CAD build for the part. Positions are in the model's coordinates, mm. A direction names the side the tool comes from. Coordinates: 2 decimals unless noted, no trailing zeros. Loops run counter-clockwise (first coordinate to the right, second up) from the corner with the lowest first, then second, coordinate; pieces in that order, holes last.
1) Saw through at A-A, the plane y = 0. Write the cut outline in (x, z).
2) Which spindle directions (+Z, -Z, +X, -X, +Y, -Y) get a long thin tool onto all of the face, cutting with end or side? Do faces 1 (the cylindrical face through (46.99, -47.15, 50.56)), 2 (the flat face through (-47.465, 0.25, 21.554)). Say none if no direction does.
3) Saw through at B-B, the plane x = 0. Write the cut outline in (y, z).
4) Saw through at C-C, the plane z = 73.5. Write the cut outline in (x, y), and give its area (3 significant figures).
5) Two-plate mould, pull along Z, no slides. Class faces 3 (the flat face through (-38, 0, 24.019)), 4 (the cylindrical face through (-47.15, 0.56, 3.01)), 5 (the cylindrical face through (-46.99, 0.56, 97.15)): +Z half, -Z half, draft (parallel to the pull), parting line (faces both ways), or undercut.
6) Pin check, flat tips, straight feed: pin 1 Ø15.5 at (y, z) = (-3.5, 53) entering from -X; pin 2 Ø15 at (x, y) = (9, -2) entering from +Z. Stop position of each tip, or through.
7) Wall check: line 1 along Y through (x, z) = (0, 84.75); line 2 along Z through (x, y) = (-30, -40.5); line 3 along X through (y, z) = (-15.5, 92.5). Give the ranges that are in metal, low to high.
```python
from build123d import *

# Parameters (mm, degrees)
SKETCH1_W           = 100
SKETCH1_H           = 100
BOSS_EXTRUDE1_DEPTH = 100
SKETCH2_R           = 25
CUT_EXTRUDE1_DEPTH  = 20
CUT_EXTRUDE3_DEPTH  = 20
CHAMFER1_SIZE       = 5
FILLET1_R           = 10
FILLET2_R           = 10
FILLET3_R           = 10


with BuildPart() as part:
    # Sketch1 → Boss-Extrude1 (new body)
    with BuildSketch(Plane.XY):
        Rectangle(SKETCH1_W, SKETCH1_H)
    extrude(amount=BOSS_EXTRUDE1_DEPTH)

    # Sketch2 → Cut-Extrude1 (cut)
    with BuildSketch(Plane.XY.offset(100)):
        Circle(SKETCH2_R)
    extrude(amount=-CUT_EXTRUDE1_DEPTH, mode=Mode.SUBTRACT)

    # Sketch6 → Cut-Extrude3 (cut)
    with BuildSketch(Plane.ZY.offset(50)):
        Polygon((69.019237886, -19.019237886), (30.980762114, 19.019237886), (24.019237886, 15), (24.019237886, -15), (50, -30), align=None)
        Polygon((50, 30), (30.980762114, 19.019237886), (69.019237886, -19.019237886), (75.980762114, -15), (75.980762114, 15), align=None)
    extrude(amount=-CUT_EXTRUDE3_DEPTH, mode=Mode.SUBTRACT)

    # Chamfer1
    chamfer1_edges = [part.edges().sort_by_distance(p)[0] for p in [
        (-50, -22.5, 37.009618943),
        (-50, -22.5, 62.990381057),
        (-50, 0, 75.980762114),
        (-50, 22.5, 62.990381057),
        (-50, 22.5, 37.009618943),
        (-50, 0, 24.019237886),
    ]]
    chamfer(chamfer1_edges, length=CHAMFER1_SIZE)

    # Fillet1
    fillet1_edges = [part.edges().sort_by_distance(p)[0] for p in [
        (-25, 0, 100),
    ]]
    fillet(fillet1_edges, radius=FILLET1_R)

    # Fillet2
    fillet2_edges = [part.edges().sort_by_distance(p)[0] for p in [
        (-50, 0, 100),
        (0, -50, 100),
        (0, -50, 0),
        (50, -50, 50),
        (-50, -50, 50),
        (-50, 50, 50),
        (0, 50, 100),
    ]]
    fillet(fillet2_edges, radius=FILLET2_R)

    # Fillet3
    # the kernel refuses this fillet: 10 mm, written as the material it takes off along each edge
    with BuildSketch(Plane(origin=(40, -40, 10), x_dir=(0, 0, -1), z_dir=(1, 0, 0))) as fillet3_piece_1_section:
        Polygon((0, 0), (FILLET3_R, 0), (FILLET3_R, -FILLET3_R), (0, -FILLET3_R), align=None)
    fillet3_piece_1 = extrude(amount=FILLET3_R, mode=Mode.PRIVATE)
    fillet3_piece_1 = fillet3_piece_1 - Plane(origin=(40, -40, 10), x_dir=(0, 0.7071067811865475, 0.7071067811865475), z_dir=(1, 0, 0)) * Sphere(FILLET3_R, mode=Mode.PRIVATE)
    add(fillet3_piece_1, mode=Mode.SUBTRACT)
    with BuildSketch(Plane(origin=(40, -40, 90), x_dir=(1, 0, 0), z_dir=(0, 0, 1))) as fillet3_piece_2_section:
        Polygon((0, 0), (FILLET3_R, 0), (FILLET3_R, -FILLET3_R), (0, -FILLET3_R), align=None)
    fillet3_piece_2 = extrude(amount=FILLET3_R, mode=Mode.PRIVATE)
    fillet3_piece_2 = fillet3_piece_2 - Plane(origin=(40, -40, 90), x_dir=(-0.7071067811865475, 0.7071067811865475, 0), z_dir=(0, 0, 1)) * Sphere(FILLET3_R, mode=Mode.PRIVATE)
    add(fillet3_piece_2, mode=Mode.SUBTRACT)
    with BuildSketch(Plane(origin=(-40, -40, 10), x_dir=(-1, 0, 0), z_dir=(0, 0, -1))) as fillet3_piece_3_section:
        Polygon((0, 0), (FILLET3_R, 0), (FILLET3_R, -FILLET3_R), (0, -FILLET3_R), align=None)
    fillet3_piece_3 = extrude(amount=FILLET3_R, mode=Mode.PRIVATE)
    fillet3_piece_3 = fillet3_piece_3 - Plane(origin=(-40, -40, 10), x_dir=(0.7071067811865475, 0.7071067811865475, 0), z_dir=(0, 0, -1)) * Sphere(FILLET3_R, mode=Mode.PRIVATE)
    add(fillet3_piece_3, mode=Mode.SUBTRACT)
    with BuildSketch(Plane(origin=(40, 40, 10), x_dir=(0, 1, 0), z_dir=(1, 0, 0))) as fillet3_piece_4_section:
        Polygon((0, 0), (FILLET3_R, 0), (FILLET3_R, -FILLET3_R), (0, -FILLET3_R), align=None)
    fillet3_piece_4 = extrude(amount=FILLET3_R, mode=Mode.PRIVATE)
    fillet3_piece_4 = fillet3_piece_4 - Plane(origin=(40, 40, 10), x_dir=(0, -0.7071067811865475, 0.7071067811865475), z_dir=(1, 0, 0)) * Sphere(FILLET3_R, mode=Mode.PRIVATE)
    add(fillet3_piece_4, mode=Mode.SUBTRACT)
    with BuildSketch(Plane(origin=(-45, -25.355339059, 75.980762114), x_dir=(-0.7071067811865476, 0, 0.7071067811865476), z_dir=(0, 1, 0))) as fillet3_piece_5_section:
        with BuildLine():
            CenterArc((FILLET3_R * 0.414213562373, FILLET3_R), FILLET3_R, 225, 45)
            Line((-FILLET3_R * 0.292893218813, FILLET3_R * 0.292893218813), (0, 0))
            Line((0, 0), (FILLET3_R * 0.414213562373, 0))
        make_face()
    fillet3_piece_5 = extrude(amount=50.710678119, mode=Mode.PRIVATE)
    fillet3_piece_5 = split(fillet3_piece_5, bisect_by=Plane(origin=(-43.280595019, -13.170460791, 75.710807016), z_dir=(0.7071067811865477, -0.6123724356957944, 0.35355339059327423)), keep=Keep.TOP, mode=Mode.PRIVATE)
    fillet3_piece_5 = split(fillet3_piece_5, bisect_by=Plane(origin=(-42.707460026, -14.659509184, 76.570509507), z_dir=(0, 0.8660254037844383, -0.5000000000000008)), keep=Keep.TOP, mode=Mode.PRIVATE)
    add(fillet3_piece_5, mode=Mode.SUBTRACT)
    with BuildSketch(Plane(origin=(-45, -25.355339059, 75.980762114), x_dir=(-0.7071067811865476, 0, 0.7071067811865476), z_dir=(0, 1, 0))) as fillet3_piece_6_section:
        with BuildLine():
            CenterArc((FILLET3_R * 0.414213562373, FILLET3_R), FILLET3_R, 225, 45)
            Line((-FILLET3_R * 0.292893218813, FILLET3_R * 0.292893218813), (0, 0))
            Line((0, 0), (FILLET3_R * 0.414213562373, 0))
        make_face()
    fillet3_piece_6 = extrude(amount=50.710678119, mode=Mode.PRIVATE)
    fillet3_piece_6 = split(fillet3_piece_6, bisect_by=Plane(origin=(-46.28634247, -15.385729384, 77.885344161), z_dir=(-0.7071067811865477, 0.6123724356957944, -0.35355339059327423)), keep=Keep.TOP, mode=Mode.PRIVATE)
    fillet3_piece_6 = split(fillet3_piece_6, bisect_by=Plane(origin=(-46.715123293, -14.271724128, 77.242172926), z_dir=(0, -0.8660254037844383, 0.5000000000000008)), keep=Keep.TOP, mode=Mode.PRIVATE)
    add(fillet3_piece_6, mode=Mode.SUBTRACT)
    with BuildSketch(Plane(origin=(-45, -25.355339059, 75.980762114), x_dir=(-0.7071067811865476, 0, 0.7071067811865476), z_dir=(0, 1, 0))) as fillet3_piece_7_section:
        with BuildLine():
            CenterArc((FILLET3_R * 0.414213562373, FILLET3_R), FILLET3_R, 225, 45)
            Line((-FILLET3_R * 0.292893218813, FILLET3_R * 0.292893218813), (0, 0))
            Line((0, 0), (FILLET3_R * 0.414213562373, 0))
        make_face()
    fillet3_piece_7 = extrude(amount=50.710678119, mode=Mode.PRIVATE)
    fillet3_piece_7 = split(fillet3_piece_7, bisect_by=Plane(origin=(-38.58008118, -5.415701855, 79.741415816), z_dir=(-0.7071067811865477, 0.6123724356957944, -0.35355339059327423)), keep=Keep.TOP, mode=Mode.PRIVATE)
    fillet3_piece_7 = split(fillet3_piece_7, bisect_by=Plane(origin=(-38.58008118, 5.415701855, 79.741415816), z_dir=(-0.7071067811865476, -0.6123724356957948, -0.3535533905932732)), keep=Keep.TOP, mode=Mode.PRIVATE)
    fillet3_piece_7 = split(fillet3_piece_7, bisect_by=Plane(origin=(-44.833595027, -10.975514643, 82.951375226), z_dir=(0, 0.8660254037844383, -0.5000000000000008)), keep=Keep.TOP, mode=Mode.PRIVATE)
    fillet3_piece_7 = split(fillet3_piece_7, bisect_by=Plane(origin=(-44.833595027, 10.975514643, 82.951375226), z_dir=(0, -0.8660254037844392, -0.49999999999999917)), keep=Keep.TOP, mode=Mode.PRIVATE)
    add(fillet3_piece_7, mode=Mode.SUBTRACT)
    with BuildSketch(Plane(origin=(-45, -25.355339059, 75.980762114), x_dir=(-0.7071067811865476, 0, 0.7071067811865476), z_dir=(0, 1, 0))) as fillet3_piece_8_section:
        with BuildLine():
            CenterArc((FILLET3_R * 0.414213562373, FILLET3_R), FILLET3_R, 225, 45)
            Line((-FILLET3_R * 0.292893218813, FILLET3_R * 0.292893218813), (0, 0))
            Line((0, 0), (FILLET3_R * 0.414213562373, 0))
        make_face()
    fillet3_piece_8 = extrude(amount=50.710678119, mode=Mode.PRIVATE)
    fillet3_piece_8 = split(fillet3_piece_8, bisect_by=Plane(origin=(-43.280595019, 13.170460791, 75.710807016), z_dir=(0.7071067811865476, 0.6123724356957948, 0.3535533905932732)), keep=Keep.TOP, mode=Mode.PRIVATE)
    fillet3_piece_8 = split(fillet3_piece_8, bisect_by=Plane(origin=(-42.707460026, 14.659509184, 76.570509507), z_dir=(0, -0.8660254037844392, -0.49999999999999917)), keep=Keep.TOP, mode=Mode.PRIVATE)
    add(fillet3_piece_8, mode=Mode.SUBTRACT)
    with BuildSketch(Plane(origin=(-45, -25.355339059, 75.980762114), x_dir=(-0.7071067811865476, 0, 0.7071067811865476), z_dir=(0, 1, 0))) as fillet3_piece_9_section:
        with BuildLine():
            CenterArc((FILLET3_R * 0.414213562373, FILLET3_R), FILLET3_R, 225, 45)
            Line((-FILLET3_R * 0.292893218813, FILLET3_R * 0.292893218813), (0, 0))
            Line((0, 0), (FILLET3_R * 0.414213562373, 0))
        make_face()
    fillet3_piece_9 = extrude(amount=50.710678119, mode=Mode.PRIVATE)
    fillet3_piece_9 = split(fillet3_piece_9, bisect_by=Plane(origin=(-46.28634247, 15.385729384, 77.885344161), z_dir=(-0.7071067811865476, -0.6123724356957948, -0.3535533905932732)), keep=Keep.TOP, mode=Mode.PRIVATE)
    fillet3_piece_9 = split(fillet3_piece_9, bisect_by=Plane(origin=(-46.715123293, 14.271724128, 77.242172926), z_dir=(0, 0.8660254037844392, 0.49999999999999917)), keep=Keep.TOP, mode=Mode.PRIVATE)
    add(fillet3_piece_9, mode=Mode.SUBTRACT)
    with BuildSketch(Plane(origin=(40, 50, 0), x_dir=(0, 0, 1), z_dir=(-1, 0, 0)), Plane(origin=(50, -40, 0), x_dir=(0, 0, 1), z_dir=(0, 1, 0)), Plane(origin=(50, 50, 10), x_dir=(0, -1, 0), z_dir=(0, 0, 1)), Plane(origin=(50, -40, 100), x_dir=(-1, 0, 0), z_dir=(0, 1, 0))) as fillet3_piece_10:
        with BuildLine():
            CenterArc((FILLET3_R, -FILLET3_R), FILLET3_R, 90, 90)
            Line((0, -FILLET3_R), (0, 0))
            Line((0, 0), (FILLET3_R, 0))
        make_face()
    extrude(amount=80, mode=Mode.SUBTRACT)
    with BuildSketch(Plane(origin=(-50, 40, 0), x_dir=(1, 0, 0), z_dir=(0, -1, 0))) as fillet3_piece_11:
        with BuildLine():
            CenterArc((FILLET3_R, FILLET3_R), FILLET3_R, 180, 90)
            Line((0, FILLET3_R), (0, 0))
            Line((0, 0), (FILLET3_R, 0))
        make_face()
    extrude(amount=80, mode=Mode.SUBTRACT)
    with BuildSketch(Plane(origin=(-40, 40, 0), x_dir=(-1, 0, 0), z_dir=(0, -1, 0))) as fillet3_piece_12:
        with BuildLine():
            CenterArc((10 - FILLET3_R, -FILLET3_R), FILLET3_R, 0, 90)
            Line((10, -FILLET3_R), (10, 0))
            Line((10, 0), (10 - FILLET3_R, 0))
        make_face()
    revolve(axis=Axis((-40, 40, 0), (0, 0, -1)), revolution_arc=90, mode=Mode.SUBTRACT)
    with BuildSketch(Plane(origin=(50, 40, 90), x_dir=(0, 0, 1), z_dir=(0, -1, 0))) as fillet3_piece_13:
        with BuildLine():
            CenterArc((10 - FILLET3_R, FILLET3_R), FILLET3_R, 270, 90)
            Line((10, FILLET3_R), (10, 0))
            Line((10, 0), (10 - FILLET3_R, 0))
        make_face()
    revolve(axis=Axis((50, 40, 90), (-1, 0, 0)), revolution_arc=90, mode=Mode.SUBTRACT)


solid = part.part
```
Data:
1. outline: (-50, 10) arc R10 ccw to (-40, 0) - (40, 0) arc R10 ccw to (50, 10) - (50, 90) arc R10 ccw to (40, 100) - (35, 100) arc R10 ccw to (25, 90) - (25, 80) - (-25, 80) - (-25, 90) arc R10 ccw to (-35, 100) - (-40, 100) arc R10 ccw to (-50, 90) - (-50, 80.98) - (-47.93, 78.91) arc R10 ccw to (-40.86, 75.98) - (-30, 75.98) - (-30, 24.02) - (-45, 24.02) - (-50, 19.02) - close
2. face 1: +Z, -Z, +X, -Y
2. face 2: -X
3. outline: (-50, 10) arc R10 ccw to (-40, 0) - (40, 0) arc R10 ccw to (50, 10) - (50, 90) arc R10 ccw to (40, 100) - (35, 100) arc R10 ccw to (25, 90) - (25, 80) - (-25, 80) - (-25, 90) arc R10 ccw to (-35, 100) - (-40, 100) arc R10 ccw to (-50, 90) - close
4. outline: (-50, -40) arc R10 ccw to (-40, -50) - (40, -50) arc R10 ccw to (50, -40) - (50, 40) arc R10 ccw to (40, 50) - (-40, 50) arc R10 ccw to (-50, 40) - (-50, 22.21) - (-45, 16.43) - (-30, 16.43) - (-30, -16.43) - (-45, -16.43) - (-50, -22.21) - close
4. area: 9,230 mm2
5. face 3: undercut
5. face 4: -Z half
5. face 5: +Z half
6. pin 1: stops at x = -30
6. pin 2: stops at z = 80
7. line 1: y = -50 to -25, 25 to 50
7. line 2: z = 0.01 to 99.99
7. line 3: x = -49.68 to -20.02, 20.02 to 49.68
